Design review of the part built by this model. Coordinates are the model's own, in mm. A direction names the side the tool comes from. Coordinates: 2 decimals unless noted, no trailing zeros. Loops run counter-clockwise (first coordinate to the right, second up) from the corner with the lowest first, then second, coordinate; pieces in that order, holes last.
Q1. Add section C-C on y = 9. Give the boundary of the cut face in (x, z), and give its area (3 significant figures).
Q2. Wall thickness on probe 1 along X at (y, z) = (30.5, 0); probe 2 along Z at (x, y) = (0, 24): over which ranges is each line inside the solid? List them lowest first.
Q3. For P1, Ø1.5, axis at y = 41.5, z = -13, coming from the +X side; P2, Ø1, axis at y = 23.5, z = 9.5, coming from the -X side; P3, Ø1.5, axis at x = -30, z = -60, coming from the +Y side; P4, Ø10, axis at y = 42, z = -7.5, coming from the +X side, all flat-tipped, find the tip position at first contact; note any pin that passes through.
Q4. Machinability: for faces 5 (the face through (-55.351, 25.044, 42.442)), 6 (the face through (16.04, 23.21, -72.24)), which of the approach directions +Z, -Z, +X, -X, +Y, -Y give a long, thin tool a straight path to every point of the face, cutting with its end or side? Answer none if there is none.
Q5. Draft analysis for pull direction Y (two halves, no side actions). For faces 1 (the face through (16.04, 38.31, -72.24)), 2 (the face through (-76.176, 4.087, -3.353)), 3 (the face through (34, 50.8, 62)), 4 (the face through (54.29, 0, -44.05)), state which applies: released by +Y, released by -Y, zero draft, split by the parting line, or undercut.
```python
from build123d import *

# Parameters (mm, degrees)
SKETCH1_R           = 76.25
SKETCH1_R_2         = 69.75
BOSS_EXTRUDE1_DEPTH = 50.8
CHAMFER1_SIZE       = 2.5


with BuildPart() as part:
    # Sketch1 → Boss-Extrude1 (new body)
    with BuildSketch(Plane(origin=(0, 0, 0), x_dir=(1, 0, 0), z_dir=(0, 1, 0))):
        Circle(SKETCH1_R)
        Circle(SKETCH1_R_2, mode=Mode.SUBTRACT)
    extrude(amount=BOSS_EXTRUDE1_DEPTH)

    # Sketch2 → Cut-Revolve1 (revolve, cut)
    with BuildSketch(Plane.XY):
        Polygon((-76.25, 40.8), (-76.25, 35.72), (-74, 34.901066973), (-74, 41.618933027), align=None)
        Polygon((-74, 26.618933027), (-74, 19.901066973), (-76.25, 20.72), (-76.25, 25.8), align=None)
        Polygon((-74, 11.618933027), (-74, 4.901066973), (-76.25, 5.72), (-76.25, 10.8), align=None)
    revolve(axis=Axis((0, 0, 0), (0, 1, 0)), mode=Mode.SUBTRACT)

    # Chamfer1
    chamfer1_edges = [part.edges().sort_by_distance(p)[0] for p in [
        (-76.25, 0, 0),
    ]]
    chamfer(chamfer1_edges, length=CHAMFER1_SIZE)


solid = part.part
```
Entries:
1. outline: circle Ø148 at (0, 0); hole circle Ø139.5 at (0, 0)
1. area: 1,920 mm2
2. probe 1: x = -76.25 to -69.75, 69.75 to 76.25
2. probe 2: z = -74 to -69.75, 69.75 to 74
3. P1: stops at x = 75.26
3. P2: stops at x = -73.45
3. P3: passes through
3. P4: stops at x = 76.21
4. face 5: +Y, -Y
4. face 6: none
5. face 1: undercut
5. face 2: zero draft
5. face 3: released by +Y
5. face 4: released by -Y
